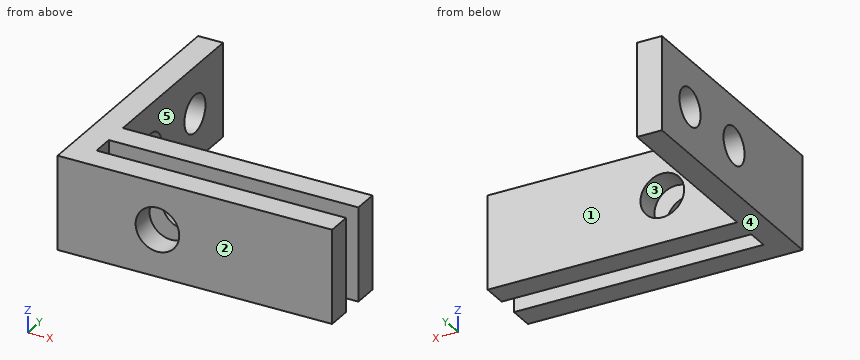
```python
from build123d import *

# Parameters (mm, degrees)
SKETCH1_W           = 7.5
SKETCH1_H           = 20
BOSS_EXTRUDE2_DEPTH = 2
SKETCH2_W           = 7.5
SKETCH2_H           = 1.98347932
BOSS_EXTRUDE3_DEPTH = 20
SKETCH3_W           = 7.5
SKETCH3_H           = 2
BOSS_EXTRUDE4_DEPTH = 20
SKETCH5_R           = 1.5
CUT_EXTRUDE1_DEPTH  = 20
SKETCH6_R           = 1.75
CUT_EXTRUDE2_DEPTH  = 10


with BuildPart() as part:
    # Sketch1 → Boss-Extrude2 (new body)
    with BuildSketch(Plane(origin=(0, 0, 0), x_dir=(0, 0, -1), z_dir=(1, 0, 0))):
        with Locations((3.009581882, -0.975609756)):
            Rectangle(SKETCH1_W, SKETCH1_H)
    extrude(amount=BOSS_EXTRUDE2_DEPTH)

    # Sketch2 → Boss-Extrude3 (add)
    with BuildSketch(Plane(origin=(2, 0, 0), x_dir=(0, 0, -1), z_dir=(1, 0, 0))):
        with Locations((3.009581882, -9.983870096)):
            Rectangle(SKETCH2_W, SKETCH2_H)
    extrude(amount=BOSS_EXTRUDE3_DEPTH)

    # Sketch3 → Boss-Extrude4 (add)
    with BuildSketch(Plane(origin=(2, 0, 0), x_dir=(0, 0, -1), z_dir=(1, 0, 0))):
        with Locations((3.009581882, -6.242130436)):
            Rectangle(SKETCH3_W, SKETCH3_H)
    extrude(amount=BOSS_EXTRUDE4_DEPTH)

    # Sketch5 → Cut-Extrude1 (cut)
    with BuildSketch(Plane(origin=(2, 0, 0), x_dir=(0, 0, -1), z_dir=(1, 0, 0))):
        with Locations((3.009581882, 5.024390244)):
            Circle(SKETCH5_R)
        with Locations((3.096458319, -1.242130436)):
            Circle(SKETCH5_R)
    extrude(amount=-CUT_EXTRUDE1_DEPTH, mode=Mode.SUBTRACT)

    # Sketch6 → Cut-Extrude2 (cut)
    with BuildSketch(Plane(origin=(0, -5.242130436, 0), x_dir=(1, 0, 0), z_dir=(0, 1, 0))):
        with Locations((8, 3.009581882)):
            Circle(SKETCH6_R)
    extrude(amount=-CUT_EXTRUDE2_DEPTH, mode=Mode.SUBTRACT)


solid = part.part
```
Verification items for the finished model (mm, model axes). Face numbers are marked on the shaded views. A direction names the side the tool comes from. Coordinates: 2 decimals unless noted, no trailing zeros. Order: outer loops, then holes, each group sorted by start corner. A loop starts at its lowest first (then second) coordinate and runs counter-clockwise, first axis right, second up. Notation, with made-up numbers: (-8.75, -25) - (10.25, -25) arc R20 cw to (10.25, -14) - close; hole circle Ø5 at (-28.75, 63.5). An arc over 180 degrees is marked (long way). Return JSON: item names as keys, results as strings.
(1) Thickness scan on line 1 along Z through (x, y) = (8, -6.8); line 2 along Y through (x, z) = (13.25, 0); line 3 along X through (y, z) = (-0.5, 0). Record the ranges inside material, lowest first.
Filled sheet:
{"line 1": "z = -6.76 to -4.76, -1.26 to 0.74", "line 2": "y = -10.98 to -8.99, -7.24 to -5.24", "line 3": "x = 0 to 2"}
(2) Mould release check, pull along X, two halves, no side actions. Record for the marked faces 3, 4 and 5: pulls with the +X half, pulls with the -X half, needs draft (parallel to the pull), parting line crosses it, or undercut.
Filled sheet:
{"face 3": "undercut", "face 4": "needs draft", "face 5": "pulls with the +X half"}
(3) Section check A-A, the plane x = 3. Record the cut outline in (y, z).
Filled sheet:
{"outline": "(-10.98, -6.76) - (-8.99, -6.76) - (-8.99, 0.74) - (-10.98, 0.74) - close; (-7.24, -6.76) - (-5.24, -6.76) - (-5.24, 0.74) - (-7.24, 0.74) - close"}
(4) Section check C-C, the plane x = 8. Record the cut outline in (y, z).
Filled sheet:
{"outline": "(-10.98, -6.76) - (-8.99, -6.76) - (-8.99, -4.76) - (-10.98, -4.76) - close; (-10.98, -1.26) - (-8.99, -1.26) - (-8.99, 0.74) - (-10.98, 0.74) - close; (-7.24, -6.76) - (-5.24, -6.76) - (-5.24, -4.76) - (-7.24, -4.76) - close; (-7.24, -1.26) - (-5.24, -1.26) - (-5.24, 0.74) - (-7.24, 0.74) - close"}
(5) Access from +Z, -Z, +X, -X, +Y, -Y to the whole of each face (thin tool, end or side, straight path). Record for the marked faces 1 and 2.
Filled sheet:
{"face 1": "+Z, -Z, +X, +Y", "face 2": "+Z, -Z, +X, -X, -Y"}
(6) Section check B-B, the plane y = 0. Record the cut outline in (x, z), and give its area (3 significant figures).
Filled sheet:
{"outline": "(0, -6.76) - (2, -6.76) - (2, -3.94) - (0, -3.94) - close; (0, -2.26) - (2, -2.26) - (2, 0.74) - (0, 0.74) - close", "area": "11.6 mm^2"}
(7) Go/stop test with flat-tipped pins: pin 1 (2 mm diameter, centred on x = 14, z = -4, fed in from +Y); pin 2 (4 mm diameter, centred on y = 0.5, z = -2, fed in from +X). Record where each tip stops, or that it passes through.
Filled sheet:
{"pin 1": "stops at y = -5.24", "pin 2": "stops at x = 2"}
(8) Section check D-D, the plane z = -5.5. Record the cut outline in (x, y).
Filled sheet:
{"outline": "(0, -10.98) - (22, -10.98) - (22, -8.99) - (2, -8.99) - (2, -7.24) - (22, -7.24) - (22, -5.24) - (2, -5.24) - (2, 9.02) - (0, 9.02) - close"}
